Autodesk Inventor part; units mm, degrees
ref_plane "YZ Plane" through (0, 0, 0) normal (1, 0, 0) x (0, 1, 0)
ref_plane "XZ Plane" through (0, 0, 0) normal (0, 1, 0) x (-1, 0, 0)
ref_plane "XY Plane" through (0, 0, 0) normal (0, 0, 1) x (1, 0, 0)
sketch "Sketch1" plane through (0, 0, 0) normal (0, 0, 1) x (1, 0, 0)
  line L0 (0, 0) -> (-35, 0)
  line L1 (0, 0) -> (0, -20)
  line L2 (0, -20) -> (-40, -20)
  arc A0 (-35, 0) -> (-40, -20) centre (-15.404, -15.524) ccw
  dimension "d0" = 35
  dimension "d1" = 20
  dimension "d2" = 40
  dimension "d3" = 25
revolve "Revolution1" add sketch "Sketch1" angle 360 about axis through (0, 0, 0) along (0, -1, 0)
sketch "Sketch2" plane through (0, -20, 0) normal (0, -1, 0) x (1, 0, 0)
  circle A0 centre (0, 0) radius 39.5
  dimension "d5" = 79
extrude "Extrusion1" add sketch "Sketch2" along normal blind 1
sketch "Sketch3" plane through (0, 0, 0) normal (1, 0, 0) x (0, 1, 0)
  line L0 (-21, 39.5) -> (-21, -39.5)
  line L1 (-21, 0) -> (-21, 40)
  line L2 (-21, 0) -> (-41, 0)
  line L3 (-41, 0) -> (-41, 42)
  arc A0 (-21, 40) -> (-41, 42) centre (-34.5432, 5.5677) ccw
  point P0 (0, 0)
  dimension "d8" = 40
  dimension "d9" = 20
  dimension "d10" = 42
  dimension "d11" = 37
revolve "Revolution2" add sketch "Sketch3" angle 360 about axis through (0, -21, 0) along (0, -1, 0)
sketch "Sketch4" plane through (0, -41, 0) normal (0, -1, 0) x (1, 0, 0)
  circle A0 centre (0, 0) radius 41.25
  dimension "d13" = 82.5
extrude "Extrusion2" add sketch "Sketch4" along normal blind 0.7
sketch "Sketch5" plane through (0, -41.7, 0) normal (0, -1, 0) x (1, 0, 0)
  circle A0 centre (0, 0) radius 42
  dimension "d16" = 84
extrude "Extrusion3" add sketch "Sketch5" along normal blind 7
sketch "Sketch6" plane through (0, -48.7, 0) normal (0, -1, 0) x (1, 0, 0)
  circle A0 centre (0, 0) radius 35
  dimension "d19" = 70
extrude "Extrusion4" add sketch "Sketch6" along normal blind 3
sketch "Sketch7" plane through (0, -48.7, 0) normal (0, -1, 0) x (1, 0, 0)
  circle A0 centre (0, 0) radius 35 construction
  line L0 (0, -35) -> (0, -42) construction
  circle A1 centre (0, 0) radius 42 construction
  circle A2 centre (0, -38.5) radius 2.25
  dimension "d22" = 4.5
extrude "Extrusion5" add sketch "Sketch7" along normal blind 2.7
sketch "Sketch8" plane through (0, -51.4, -38.5) normal (0, -1, 0) x (1, 0, 0)
  circle A0 centre (0, 0) radius 2.25
  circle A1 centre (0, 0) radius 1.55
  point P0 (0, 38.5)
  dimension "d25" = 0.7
extrude "Extrusion6" cut sketch "Sketch8" against normal blind 0.5 contours A1
pattern_circular "Circular Pattern1" count 12 over 360 about axis through (0, -48.7, 0) along (0, -1, 0) of "Extrusion5", "Extrusion6"
sketch "Sketch9" plane through (0, 0, 0) normal (0, 1, 0) x (1, 0, 0)
  line L0 (-10, -20) -> (10, -20)
  line L1 (10, -20) -> (10, 20)
  line L2 (10, 20) -> (-10, 20)
  line L3 (-10, 20) -> (-10, -20)
  line L4 (-10, -20) -> (10, 20) construction
  line L5 (10, -20) -> (-10, 20) construction
  point P0 (0, 0)
  dimension "d31" = 20
  dimension "d32" = 40
extrude "Extrusion7" add sketch "Sketch9" along normal blind 42
sketch "Sketch10" plane through (10, 0, 20) normal (1, 0, 0) x (0, 0, -1)
  line L0 (0, 42) -> (40, 42)
  circle A0 centre (20, 42) radius 20
  point P0 (20, 0)
extrude "Extrusion8" add sketch "Sketch10" against normal up to surface (20 mm away)
sketch "Sketch11" plane through (-10, 0, -20) normal (-1, 0, 0) x (0, 0, 1)
  arc A0 (40, 42) -> (0, 42) centre (20, 42) ccw
  circle A1 centre (20, 42) radius 15
  point P0 (20, 0)
  dimension "d37" = 30
extrude "Extrusion9" add sketch "Sketch11" along normal blind 20
mirror "Mirror1" about plane through (0, 0, 0) normal (1, 0, 0) of "Extrusion9"
sketch "Sketch12" plane through (0, -51.7, 0) normal (0, -1, 0) x (1, 0, 0)
  circle A0 centre (0, 0) radius 15
  dimension "d40" = 30
extrude "Extrusion10" add sketch "Sketch12" along normal blind 20
Geometry: final body of the model. Coordinates: model frame, mm. A direction names the side the tool comes from. Coordinates: 2 decimals unless noted, no trailing zeros. Loops run counter-clockwise (first coordinate to the right, second up) from the corner with the lowest first, then second, coordinate; pieces in that order, holes last. Notation, with made-up numbers: M -29.75,52 L -10.75,52 A15 cw -10.75,61 Z; hole C 63.5,54.5 d7. An arc over 180 degrees is marked long. Put each result on its own line as item: value.
(1) Material intervals for probe 1 along Z at (x, y) = (0, -51.1); probe 2 along Z at (x, y) = (38.5, -51.15); probe 3 along Y at (x, z) = (12.5, 16.5), sorted ascending.
Answer sheet:
probe 1: z = -40.75 to -40.05, -36.95 to -36.25, -35 to 35, 36.25 to 36.95, 40.05 to 40.75
probe 2: z = -2.25 to -1.55, 1.55 to 2.25
probe 3: y = -51.7 to 0
(2) Cut plane B-B on y = -56.5. Return the cut outline in (x, z).
Answer sheet:
outline: C 0,0 d30
(3) Cut plane A-A on y = 30. Return the cut outline in (x, z).
Answer sheet:
outline: M -30,-9 L -10,-9 L -10,-20 L 10,-20 L 10,-9 L 30,-9 L 30,9 L 10,9 L 10,20 L -10,20 L -10,9 L -30,9 Z
(4) Draft query along Z for faces 5 (the face through (-17.02, -50.03, -33.63)), 6 (the face through (30, 42, 0)), 7 (the face through (0, 21, 20)). Return one class per face: pulls with the +Z half, pulls with the -Z half, needs draft (parallel to the pull), parting line crosses it, or undercut.
Answer sheet:
face 5: undercut
face 6: needs draft
face 7: pulls with the +Z half
(5) First-contact query: pin 1 (1.9 mm diameter, centred on x = -19.25, z = -33.34, fed in from -Y); pin 2 (3 mm diameter, centred on y = 7.5, z = -15.5, fed in from +X); pin 3 (5 mm diameter, centred on x = 22, y = -46, fed in from -Z). Flat tips, straight axial feed; report the tip coordinate or a pass-through.
Answer sheet:
pin 1: stops at y = -50.9
pin 2: stops at x = 10
pin 3: stops at z = -37.2
(6) Access query for faces 1 (the face through (40, -51.4, -1)), 2 (the face through (-19, -50.9, 33)), 3 (the face through (-19.86, 27.128, -1.953)), 4 (the face through (-15, 0, 0)). Directions: +Z, -Z, +X, -X, +Y, -Y. A direction counts if a zero-diameter tool reaches every point of the face in a straight line with its end or side. Return the directions, or none.
Answer sheet:
face 1: +Z, -Z, +X, -Y
face 2: -Y
face 3: -X
face 4: none
